Input: part model. Units: mm. Frame: model coordinates. A direction names the side the tool comes from. Round coordinates to 2 decimals unless told otherwise and drop trailing zeros. Loops run counter-clockwise (first coordinate to the right, second up) from the corner with the lowest first, then second, coordinate; pieces in that order, holes last.
(1) Cut plane A-A, the plane y = 0. Output: boundary loops of the cut face in (x, z), and give its area (3 significant figures).
(2) Cut plane D-D, the plane y = 29. Output: boundary loops of the cut face in (x, z).
(3) Cut plane B-B, the plane x = -36. Output: boundary loops of the cut face in (y, z), and give its area (3 significant figures).
(4) Access query for faces 1 (the face through (-30, 35, -0.5)), 2 (the face through (-8.828, -48.738, 0.007)). Directions: +Z, -Z, +X, -X, +Y, -Y. A direction counts if a zero-diameter tool reaches every point of the face in a straight line with its end or side. Return the directions, or none.
(5) Line query: line 1 (X direction, y = -34, z = 0.4); line 2 (X direction, y = -35, z = 0.25); line 3 (X direction, y = -27, z = -0.2). Output: solid intervals per line, ascending.
(6) Draft query along X for faces 3 (the face through (4.55, -49.32, -0.01)), 4 (the face through (39.8, 34.5, 0)), 5 (the face through (-30, 35, 0.5)), 6 (the face through (26.76, -51.46, 0.01)). Return one class per face: released by +X, released by -X, zero draft, split by the parting line, or undercut.
(7) Cut plane C-C, the plane z = -0.2. Output: boundary loops of the cut face in (x, y).
Autodesk Inventor part; units mm, degrees
ref_plane "YZ Plane" through (0, 0, 0) normal (1, 0, 0) x (0, 1, 0)
ref_plane "XZ Plane" through (0, 0, 0) normal (0, 1, 0) x (-1, 0, 0)
ref_plane "XY Plane" through (0, 0, 0) normal (0, 0, 1) x (1, 0, 0)
sketch "Эскиз1" plane through (0, 0, 0) normal (0, 0, 1) x (1, 0, 0)
  circle A0 centre (0, 0) radius 58
  arc A1 (6.8914, -45.228) -> (-10.8071, -44.4552) centre (0, 0) ccw
  circle A2 centre (0, 0) radius 51 construction
  circle A3 centre (36.0624, 36.0624) radius 4.05
  circle A4 centre (-36.0624, 36.0624) radius 4.05
  circle A5 centre (-36.0624, -36.0624) radius 4.05
  circle A6 centre (36.0624, -36.0624) radius 4.05
  line L0 (0, 0) -> (0, 51) construction
  line L1 (0, 0) -> (36.0624, 36.0624) construction
  line L2 (0, 0) -> (-36.0624, 36.0624) construction
  line L3 (0, 0) -> (36.0624, -36.0624) construction
  line L4 (0, 0) -> (-36.0624, -36.0624) construction
  line L5 (0, 0) -> (0, -51) construction
  line L6 (0, 0) -> (-4.4449, -50.8059) construction
  arc A7 (-10.8071, -44.4552) -> (-4.4449, -50.8059) centre (-3.8349, -43.8326) ccw
  arc A8 (0, -51) -> (6.8914, -45.228) centre (0, -44) ccw
  arc A9 (-4.4449, -50.8059) -> (0, -51) centre (0, 0) ccw
  dimension "d2" = 102
  dimension "d0" = 116
  dimension "d1" = 91.5
  dimension "d3" = 8.1
  dimension "d4" = 45
  dimension "d5" = 90
  dimension "d6" = 90
  dimension "d7" = 45
  dimension "d8" = 5
  dimension "d9" = 7
  dimension "d10" = 7
extrude "Выдавливание1" add sketch "Эскиз1" along normal mid plane 1
properties part number "75. Прокладка крышки"
Reported:
1. outline: (-58, -0.5) - (-45.75, -0.5) - (-45.75, 0.5) - (-58, 0.5) - close; (45.75, -0.5) - (58, -0.5) - (58, 0.5) - (45.75, 0.5) - close
1. area: 24.5 mm2
2. outline: (-50.23, -0.5) - (-35.38, -0.5) - (-35.38, 0.5) - (-50.23, 0.5) - close; (35.38, -0.5) - (50.23, -0.5) - (50.23, 0.5) - (35.38, 0.5) - close
3. outline: (-45.48, -0.5) - (-40.11, -0.5) - (-40.11, 0.5) - (-45.48, 0.5) - close; (-32.01, -0.5) - (-28.23, -0.5) - (-28.23, 0.5) - (-32.01, 0.5) - close; (28.23, -0.5) - (32.01, -0.5) - (32.01, 0.5) - (28.23, 0.5) - close; (40.11, -0.5) - (45.48, -0.5) - (45.48, 0.5) - (40.11, 0.5) - close
3. area: 18.3 mm2
4. face 1: -Z, +X, -X, +Y, -Y
4. face 2: +Z, -Z
5. line 1: x = -46.99 to -39.55, -32.58 to -30.61, 30.61 to 32.58, 39.55 to 46.99
5. line 2: x = -46.25 to -39.97, -32.15 to -29.46, 29.46 to 32.15, 39.97 to 46.25
5. line 3: x = -51.33 to -36.93, 36.93 to 51.33
6. face 3: undercut
6. face 4: undercut
6. face 5: zero draft
6. face 6: split by the parting line
7. outline: circle Ø116 at (0, 0); hole circle Ø8.1 at (-36.06, -36.06); hole circle Ø8.1 at (-36.06, 36.06); hole (-10.81, -44.46) arc R7 ccw to (-4.44, -50.81) arc R51.02 ccw to (0, -51) arc R7 ccw to (6.89, -45.23) arc R45.75 ccw (long way) to start; hole circle Ø8.1 at (36.06, -36.06); hole circle Ø8.1 at (36.06, 36.06)
